from build123d import *

# Parameters (mm, degrees)
SKETCH1_R            = 45
SKETCH1_R_2          = 33.75
BOSS_EXTRUDE1_DEPTH  = 92.5
SKETCH4_W            = 10
SKETCH4_H            = 8.25
CUT_EXTRUDE1_DEPTH   = 120.278560521
M3_CLEARANCE_HOLE1_D = 3.4
CIRPATTERN1_COUNT    = 6


with BuildPart() as part:
    # Sketch1 → Boss-Extrude1 (new, symmetric)
    with BuildSketch(Plane.XY):
        Circle(SKETCH1_R)
        Circle(SKETCH1_R_2, mode=Mode.SUBTRACT)
    extrude(amount=BOSS_EXTRUDE1_DEPTH, both=True)

    # Sketch2 → Cut-Revolve1 (revolve, cut)
    with BuildSketch(Plane(origin=(0, 0, 0), x_dir=(1, 0, 0), z_dir=(0, 1, 0)), mode=Mode.PRIVATE) as cut_revolve1_sk:
        Polygon((0, -92.5), (0, 92.5), (-38.25, 92.5), (-38.25, 86.15), (-36.25, 86.15), (-36.25, -13.85), (-38.25, -13.85), (-38.25, -92.5), align=None)
    revolve(cut_revolve1_sk.sketch.rotate(Axis((0, 0, 92.5), (0, 0, -1)), 180), axis=Axis((0, 0, 92.5), (0, 0, -1)), mode=Mode.SUBTRACT)

    # Sketch4 → Revolve1 (revolve)
    with BuildSketch(Plane(origin=(0, 0, 0), x_dir=(0, 0, -1), z_dir=(1, 0, 0)), mode=Mode.PRIVATE) as revolve1_sk:
        with Locations((-57.5, 49.125)):
            Rectangle(SKETCH4_W, SKETCH4_H)
        with Locations((57.5, 49.125)):
            Rectangle(SKETCH4_W, SKETCH4_H)
    revolve(revolve1_sk.sketch.rotate(Axis((0, 0, -92.5), (0, 0, 1)), 90), axis=Axis((0, 0, -92.5), (0, 0, 1)))

    # Sketch3 → Cut-Extrude1 (cut, through all)
    with BuildSketch(Plane(origin=(0, 0, 0), x_dir=(1, 0, 0), z_dir=(0, 1, 0))):
        with BuildLine():
            Line((-12.5, -27.5), (12.5, -27.5))
            ThreePointArc((12.5, -27.5), (22.5, -37.5), (12.5, -47.5))
            Line((12.5, -47.5), (-12.5, -47.5))
            ThreePointArc((-12.5, -47.5), (-22.5, -37.5), (-12.5, -27.5))
        make_face()
    extrude(amount=CUT_EXTRUDE1_DEPTH, mode=Mode.SUBTRACT)

    # M3 Clearance Hole1 (through all)
    with Locations(Plane.XY.offset(62.5)):
        with Locations((0, 49.125)):
            m3_clearance_hole1 = Hole(M3_CLEARANCE_HOLE1_D / 2)

    # CirPattern1: M3 Clearance Hole1 ×6 about axis
    cirpattern1_axis = Axis((0, 0, 0), (0, 0, 1))
    for i in range(1, CIRPATTERN1_COUNT):
        add(m3_clearance_hole1.rotate(cirpattern1_axis, i * 360 / CIRPATTERN1_COUNT), mode=Mode.SUBTRACT)


solid = part.part
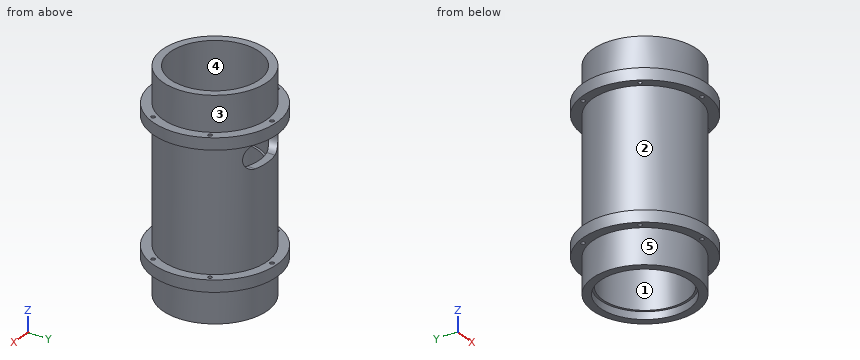
Verification items for the finished model (mm, model axes). Face numbers are marked on the shaded views. A direction names the side the tool comes from. Coordinates: 2 decimals unless noted, no trailing zeros. Write each loop counter-clockwise with the first axis right and the second up, starting at its lowest first coordinate (ties: lowest second). Pieces come first, ordered by that corner, then holes. Notation, with made-up numbers: M 1.25,-20.5 L 10.25,-20.5 A18 ccw 10.25,5.5 Z; hole C 12.25,-12.5 d1. An arc over 180 degrees is marked long. Use a Markdown table: item, result.
Q1. Set-up check for the marked faces 1, 2 and 3: record each of +Z, -Z, +X, -X, +Y, -Y from which the full face is reachable in a straight line by a thin tool's end or side.
Reply:
| item | result |
|---|---|
| face 1 | +Z, -Z |
| face 2 | none |
| face 3 | +Z |
Q2. Go/stop test with flat-tipped pins: P1, Ø4.5, axis at x = 42.54, y = -24.56, coming from the -Z side; P2, Ø2, axis at x = 40.5, z = -39, coming from the -Y side; P3, Ø2, axis at x = -33, z = 7.5, coming from the -Y side. Record where each tip stops, or that it passes through.
Reply:
| item | result |
|---|---|
| P1 | stops at z = -62.5 |
| P2 | stops at y = -21.56 |
| P3 | stops at y = -31.64 |
Q3. Thickness scan on line 1 (Y direction, x = 0, z = 57.5) (3 decimals); line 2 (Z direction, x = -20.5, y = 44.5); line 3 (X direction, y = -1.5, z = -5) (3 decimals). Record the ranges inside material, lowest first.
Reply:
| item | result |
|---|---|
| line 1 | y = -53.25 to -50.825, -47.425 to -38.25, 38.25 to 47.425, 50.825 to 53.25 |
| line 2 | z = -62.5 to -52.5, 52.5 to 62.5 |
| line 3 | x = -44.975 to -36.219, 36.219 to 44.975 |
Q4. Draft check along X on the marked faces 4 and 5. Enter one of: +X half, -X half, draft (parallel to the pull), parting line (faces both ways), or undercut.
Reply:
| item | result |
|---|---|
| face 4 | undercut |
| face 5 | parting line |
Q5. Sectioned sample at B-B, the plane z = -58. Count the separate pieces of the cut face and the enclosed holes in it, plus the area to 3 significant figures.
Reply:
| item | result |
|---|---|
| separate pieces | 1 |
| enclosed holes | 7 |
| area | 4,730 mm² |
Q6. Sectioned sample at D-D, the plane z = 7. Record the boundary of the cut face in (x, y).
Reply:
| item | result |
|---|---|
| outline | C 0,0 d90; hole C 0,0 d72.5 |
